Could you check a few things on this model? Use its own coordinates, in mm. A direction names the side the tool comes from. Coordinates: 2 decimals unless noted, no trailing zeros. Order: outer loops, then holes, each group sorted by start corner. A loop starts at its lowest first (then second) coordinate and runs counter-clockwise, first axis right, second up.
```python
from build123d import *

# Parameters (mm, degrees)
ESQUISSE1_W        = 35
ESQUISSE1_H        = 20
BOSS_EXTRU_1_DEPTH = 1.8
ESQUISSE2_W        = 35
ESQUISSE2_H        = 1.8
BOSS_EXTRU_2_DEPTH = 10.2
D_GAGEMENT_M31_D   = 3.4
D_GAGEMENT_M32_D   = 3.4


with BuildPart() as part:
    # Esquisse1 → Boss.-Extru.1 (new body)
    with BuildSketch(Plane(origin=(0, 0, 0), x_dir=(1, 0, 0), z_dir=(0, 1, 0))):
        Rectangle(ESQUISSE1_W, ESQUISSE1_H)
    extrude(amount=BOSS_EXTRU_1_DEPTH)

    # Esquisse2 → Boss.-Extru.2 (add)
    with BuildSketch(Plane(origin=(0, 1.8, 0), x_dir=(1, 0, 0), z_dir=(0, 1, 0))):
        with Locations((0, 9.1)):
            Rectangle(ESQUISSE2_W, ESQUISSE2_H)
    extrude(amount=BOSS_EXTRU_2_DEPTH)

    # Dégagement M31 (through all)
    with Locations(Plane.XY.offset(-8.2)):
        with Locations((-10.7, 6), (10.7, 6)):
            Hole(D_GAGEMENT_M31_D / 2)

    # Dégagement M32 (through all)
    with Locations(Plane(origin=(0, 1.8, 0), x_dir=(1, 0, 0), z_dir=(0, 1, 0))):
        with Locations((-10.3, -3.25), (10.3, -3.25)):
            Hole(D_GAGEMENT_M32_D / 2)


solid = part.part
```
Item 1: I need wall thicknesses on line 1 (Y direction, x = 10.7, z = -8.85); line 2 (Z direction, x = -2, y = 3.5); line 3 (Z direction, x = 10.3, y = 1.1). Which ranges of each line are inside material? Lowest first, please.
Item 2: Thinking about a two-plate mould opening in Z: for faces 3 (the face through (12, 0.9, 3.2)), 4 (the face through (0, 7, -8.2)), 5 (the face through (-9.35, 4.97, -9.11)), 6 (the face through (-9.93, 0.89, 4.91)), which applies, +Z half, -Z half, draft (parallel to the pull), parting line (faces both ways), or undercut?
Item 3: Which directions (+Z, -Z, +X, -X, +Y, -Y) give clear straight access to the entire face, cutting with the end or side of a thin tool? Please do faces 1 (the face through (0, 1.8, 1)), 2 (the face through (0, 1, 10)).
Item 4: Suppose I cut it at B-B (z = 3.25). List the corners of the cut face in (x, y) for me, and give its area (3 significant figures).
Item 5: Suppose I cut it at D-D (x = -4.5). List the corners of the cut face in (y, z) for me, and give its area (3 significant figures).
Item 6: Suppose I cut it at A-A (y = 6). List the corners of the cut face in (x, z) for me, and give its area (3 significant figures).
Item 7: For pin 1 Ø5.5 at (x, z) = (-5.5, -2) entering from +Y; pin 2 Ø2 at (x, y) = (1, 7) entering from +Z, each with a flat end and sliding along its axis, tell me the tip position at first contact or that it passes through.
Item 8: Suppose I cut it at C-C (x = -10.7). List the corners of the cut face in (y, z) for me, and give its area (3 significant figures).
Geometry results:
1. line 1: y = 0 to 4.3, 7.7 to 12
1. line 2: z = -10 to -8.2
1. line 3: z = -10 to 1.55, 4.95 to 10
2. face 3: undercut
2. face 4: +Z half
2. face 5: draft
2. face 6: undercut
3. face 1: +Z, +X, -X, +Y
3. face 2: +Z, +X, -X, +Y, -Y
4. outline: (-17.5, 0) - (-12, 0) - (-12, 1.8) - (-17.5, 1.8) - close; (-8.6, 0) - (8.6, 0) - (8.6, 1.8) - (-8.6, 1.8) - close; (12, 0) - (17.5, 0) - (17.5, 1.8) - (12, 1.8) - close
4. area: 50.8 mm2
5. outline: (0, -10) - (12, -10) - (12, -8.2) - (1.8, -8.2) - (1.8, 10) - (0, 10) - close
5. area: 54.4 mm2
6. outline: (-17.5, -10) - (-12.4, -10) - (-12.4, -8.2) - (-17.5, -8.2) - close; (-9, -10) - (9, -10) - (9, -8.2) - (-9, -8.2) - close; (12.4, -10) - (17.5, -10) - (17.5, -8.2) - (12.4, -8.2) - close
6. area: 50.8 mm2
7. pin 1: stops at y = 1.8
7. pin 2: stops at z = -8.2
8. outline: (0, -10) - (4.3, -10) - (4.3, -8.2) - (1.8, -8.2) - (1.8, 1.6) - (0, 1.6) - close; (0, 4.9) - (1.8, 4.9) - (1.8, 10) - (0, 10) - close; (7.7, -10) - (12, -10) - (12, -8.2) - (7.7, -8.2) - close
8. area: 42.3 mm2
